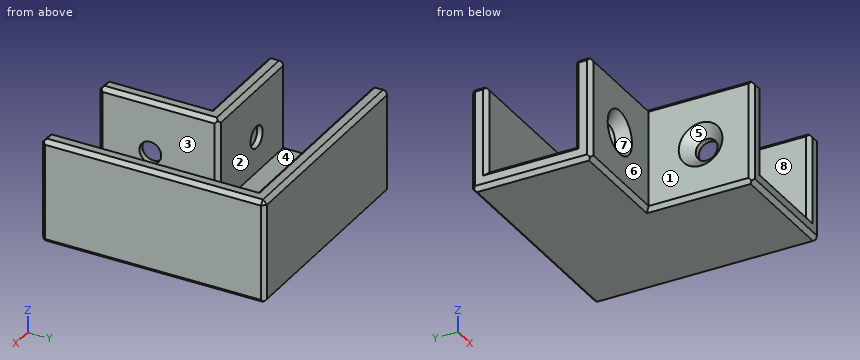
from build123d import *

# Parameters (mm, degrees)
F0_W           = 22
F0_H           = 19
F1_DEPTH       = 3
F2_W           = 3
F2_H           = 38
F2_W_2         = 19
F2_H_2         = 3
F3_DEPTH       = 16
F5_D           = 4
F5_DEPTH       = 12
F5_CSINK_D     = 8
F5_CSINK_ANGLE = 90
F5_TIP         = 1.2017212381
F7_D           = 4
F7_DEPTH       = 12
F7_CSINK_D     = 8
F7_CSINK_ANGLE = 90
F7_TIP         = 1.2017212381
F8_SIZE        = 0.75
F9_SIZE        = 0.75
F10_SIZE       = 0.75
F11_SIZE       = 0.75
F12_SIZE       = 0.75


with BuildPart() as f1:
    # F0 (on Top) → F1 (new body)
    with BuildSketch(Plane.XY):
        Polygon((0, 22), (0, 0), (19, 0), (41, 0), (41, 22), align=None)
        with Locations((30, -9.5)):
            Rectangle(F0_W, F0_H)
    extrude(amount=F1_DEPTH)

    # F2 (on face) → F3 (join)
    with BuildSketch(Plane.XY.offset(3)):
        Polygon((41, 22), (0, 22), (0, 19), (38, 19), (41, 19), align=None)
        with Locations((39.5, 0)):
            Rectangle(F2_W, F2_H)
        Polygon((22, 3), (19, 3), (19, 0), (19, -19), (22, -19), align=None)
        with Locations((9.5, 1.5)):
            Rectangle(F2_W_2, F2_H_2)
    extrude(amount=F3_DEPTH)

    # F5
    with Locations(Plane.XZ):
        with Locations((9.5, 9.5)):
            CounterSinkHole(F5_D / 2, F5_CSINK_D / 2, depth=F5_DEPTH, counter_sink_angle=F5_CSINK_ANGLE)
            with Locations((0, 0, -(F5_DEPTH + F5_TIP / 2))):  # 118° drill point
                Cone(0, F5_D / 2, F5_TIP, mode=Mode.SUBTRACT)

    # F7
    with Locations(Plane(origin=(19, 0, 0), x_dir=(0, -1, 0), z_dir=(-1, 0, 0))):
        with Locations((9.5, 9.5)):
            CounterSinkHole(F7_D / 2, F7_CSINK_D / 2, depth=F7_DEPTH, counter_sink_angle=F7_CSINK_ANGLE)
            with Locations((0, 0, -(F7_DEPTH + F7_TIP / 2))):  # 118° drill point
                Cone(0, F7_D / 2, F7_TIP, mode=Mode.SUBTRACT)

    # F8
    f8_edges = [f1.edges().sort_by_distance(p)[0] for p in [
        (19, -19, 9.5),
        (20.5, -19, 19),
        (22, -19, 11),
        (30, -19, 3),
        (38, -19, 11),
        (39.5, -19, 19),
        (41, -19, 9.5),
        (30, -19, 0),
    ]]
    chamfer(f8_edges, length=F8_SIZE)

    # F9
    f9_edges = [f1.edges().sort_by_distance(p)[0] for p in [
        (0, 22, 9.5),
        (0, 20.5, 19),
        (0, 19, 11),
        (0, 11, 3),
        (0, 3, 11),
        (0, 1.5, 19),
        (0, 0, 9.5),
        (0, 11, 0),
    ]]
    chamfer(f9_edges, length=F9_SIZE)

    # F10
    f10_edges = [f1.edges().sort_by_distance(p)[0] for p in [
        (19, -9.125, 19),
        (9.875, 0, 19),
        (11.375, 3, 19),
        (22, -7.625, 19),
        (38, 0.375, 19),
        (19.375, 19, 19),
        (20.875, 22, 19),
        (41, 1.875, 19),
        (41, 22, 9.5),
    ]]
    chamfer(f10_edges, length=F10_SIZE)

    # F11
    f11_edges = [f1.edges().sort_by_distance(p)[0] for p in [
        (22, 3, 10.625),
    ]]
    chamfer(f11_edges, length=F11_SIZE)

    # F12 (call 1 of 3: OpenCascade refuses the feature's edges together)
    f12_edges = [f1.edges().sort_by_distance(p)[0] for p in [
        (19, -9.125, 0),
        (9.875, 0, 0),
    ]]
    chamfer(f12_edges, length=F12_SIZE)

    # F12#2 (call 2 of 3)
    f12_2_edges = [f1.edges().sort_by_distance(p)[0] for p in [
        (41, 1.5, 0),
    ]]
    chamfer(f12_2_edges, length=F12_SIZE)

    # F12#3 (call 3 of 3)
    f12_3_edges = [f1.edges().sort_by_distance(p)[0] for p in [
        (20.5, 22, 0),
    ]]
    chamfer(f12_3_edges, length=F12_SIZE)


solid = f1.part
Geometry: final body of the model. Coordinates: model frame, mm. Face numbers are marked on the shaded views. A direction names the side the tool comes from. Give positions to 0.01 mm unless a question says otherwise; leave off trailing zeros. Write each loop counter-clockwise with the first axis right and the second up, starting at its lowest first coordinate (ties: lowest second). Pieces come first, ordered by that corner, then holes. Notation, with made-up numbers: M -0.5,56.5 L 44.5,56.5 A26 cw 44.5,84.5 Z; hole C 9,-0.75 d1. An arc over 180 degrees is marked long. Answer in a Markdown table with one row per item. Add a question column.
(1) Section C-C on y = -9.5. Return loops of the section in (x, z).
(2) Ray query, line 1 (X direction, y = -7, z = 4.5); line 2 (Y direction, x = 14, z = 15.5); line 3 (X direction, y = 0.5, z = 9.75). Return the intervals inside material, ascending.
(3) Section A-A on x = 9.5. Return loops of the section in (y, z), and give its area (3 significant figures).
(4) Reachability of the marked faces 1, 2, 3 and 4 from +Z, -Z, +X, -X, +Y, -Y: full face, straight path, thin tool, end or side. Return the list, or none.
(5) Section D-D on z = 3.75. Return loops of the section in (x, y), and give its area (3 significant figures).
(6) Mould query, pull axis X, two halves, no side actions, for the marked faces 5, 6, 7 and 8. Classes: +X half, -X half, draft (parallel to the pull), parting line (faces both ways), or undercut.
(7) Section B-B on z = 9.5. State how many separate pieces and enclosed holes the cut face has, and give its area (3 significant figures).
(8) First-contact query: pin 1 (8 mm diameter, centred on x = 8, y = 0.5, fed in from +Z); pin 2 (4.5 mm diameter, centred on x = 15, z = 14, fed in from -Y). Flat tips, straight axial feed; report the tip coordinate or a pass-through.
Result set:
| question | item | result |
|---|---|---|
| 1 | outline | M 19,0.75 L 19.75,0 L 40.25,0 L 41,0.75 L 41,18.25 L 40.25,19 L 38.75,19 L 38,18.25 L 38,3 L 22,3 L 22,7.5 L 21,7.5 L 19,5.5 Z; M 19,13.5 L 21,11.5 L 22,11.5 L 22,18.25 L 21.25,19 L 19.75,19 L 19,18.25 Z |
| 2 | line 1 | x = 19 to 22, 38 to 41 |
| 2 | line 2 | y = 0 to 3, 19 to 22 |
| 2 | line 3 | x = 0.25 to 6.01, 12.99 to 22, 38 to 41 |
| 3 | outline | M 0,0.75 L 0.75,0 L 21.25,0 L 22,0.75 L 22,18.25 L 21.25,19 L 19.75,19 L 19,18.25 L 19,3 L 3,3 L 3,7.5 L 2,7.5 L 0,5.5 Z; M 0,13.5 L 2,11.5 L 3,11.5 L 3,18.25 L 2.25,19 L 0.75,19 L 0,18.25 Z |
| 3 | area | 144 mm^2 |
| 4 | face 1 | +Z, -Z, -X, -Y |
| 4 | face 2 | +Z, -X |
| 4 | face 3 | +Z, -Y |
| 4 | face 4 | +Z |
| 5 | outline | M 0,0.75 L 0.75,0 L 19,0 L 19,-18.25 L 19.75,-19 L 21.25,-19 L 22,-18.25 L 22,2.25 L 21.25,3 L 0.75,3 L 0,2.25 Z; M 0,19.75 L 0.75,19 L 38,19 L 38,-18.25 L 38.75,-19 L 40.25,-19 L 41,-18.25 L 41,21.25 L 40.25,22 L 0.75,22 L 0,21.25 Z |
| 5 | area | 357 mm^2 |
| 6 | face 5 | -X half |
| 6 | face 6 | draft |
| 6 | face 7 | undercut |
| 6 | face 8 | undercut |
| 7 | separate pieces | 4 |
| 7 | enclosed holes | 0 |
| 7 | area | 325 mm^2 |
| 8 | pin 1 | stops at z = 19 |
| 8 | pin 2 | stops at y = 0 |
